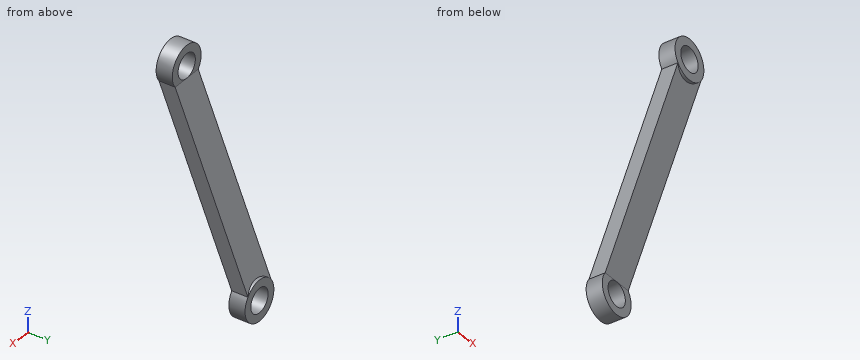
```python
from build123d import *

# Parameters (mm, degrees)
BOSS_EXTRUDE1_DEPTH = 4
SKETCH2_R           = 2.5
BOSS_EXTRUDE2_DEPTH = 2
SKETCH3_R           = 2.5
BOSS_EXTRUDE3_DEPTH = 2
SKETCH4_R           = 1.5
CUT_EXTRUDE1_DEPTH  = 28.879203719
SKETCH5_R           = 1.5
CUT_EXTRUDE2_DEPTH  = 29.587584718


with BuildPart() as part:
    # Sketch1 → Boss-Extrude1 (new body)
    with BuildSketch(Plane(origin=(0, 0, 0), x_dir=(0, 0, -1), z_dir=(1, 0, 0))):
        Polygon((0, 0), (0, 2), (22, 11), (22, 9), align=None)
    extrude(amount=BOSS_EXTRUDE1_DEPTH)

    # Sketch2 → Boss-Extrude2 (add)
    with BuildSketch(Plane(origin=(0, 0, 0), x_dir=(1, 0, 0), z_dir=(0, 1, 0))):
        with Locations((2, -1.5)):
            Circle(SKETCH2_R)
    extrude(amount=BOSS_EXTRUDE2_DEPTH)

    # Sketch3 → Boss-Extrude3 (add)
    with BuildSketch(Plane(origin=(0, 9, 0), x_dir=(-1, 0, 0), z_dir=(0, -1, 0))):
        with Locations((-2, 23.5)):
            Circle(SKETCH3_R)
    extrude(amount=-BOSS_EXTRUDE3_DEPTH)

    # Sketch4 → Cut-Extrude1 (cut, through all)
    with BuildSketch(Plane(origin=(0, 2, 0), x_dir=(1, 0, 0), z_dir=(0, 1, 0))):
        with Locations(Location((2, -1.5, 0), (0, 0, 270))):
            Circle(SKETCH4_R)
    extrude(amount=-CUT_EXTRUDE1_DEPTH, mode=Mode.SUBTRACT)

    # Sketch5 → Cut-Extrude2 (cut, through all)
    with BuildSketch(Plane(origin=(0, 11, 0), x_dir=(1, 0, 0), z_dir=(0, 1, 0))):
        with Locations(Location((2, 23.5, 0), (0, 0, 270))):
            Circle(SKETCH5_R)
    extrude(amount=-CUT_EXTRUDE2_DEPTH, mode=Mode.SUBTRACT)


solid = part.part
```
Read the model definition and answer for the solid it produces. Units are mm, in the model's axes. Round coordinates to 2 decimals unless told otherwise and drop trailing zeros. Write each loop counter-clockwise with the first axis right and the second up, starting at its lowest first coordinate (ties: lowest second). Pieces come first, ordered by that corner, then holes. Notation, with made-up numbers: M -39.75,-23 L -19.75,-23 A16 cw -19.75,-17 Z; hole C 50.25,3.5 d9. An arc over 180 degrees is marked long. One line per item, written item: value.
Q1. Flat-ended cylindrical pins translate along their axes: pin 1 Ø1.5 at (x, y) = (4, 4.5) entering from -Z; pin 2 Ø1.2 at (x, z) = (2.5, 1) entering from +Y; pin 3 Ø3 at (x, z) = (3.5, -15.5) entering from +Y; pin 4 Ø1.5 at (x, z) = (2.5, -1) entering from -Y. Find the tip coordinate at first contact, or state that the pin passes through.
Data:
pin 1: z = -12.83
pin 2: through
pin 3: y = 8.95
pin 4: y = 0
Q2. Find section C-C on y = 0.75. Write down the section's boundary in (x, z).
Data:
outline: M 0,-1.83 L 4,-1.83 L 4,0 A2.5 ccw long 0,0 Z; hole C 2,1.5 d3
Q3. Find section A-A on z = 1.5. Write down the section's boundary in (x, y).
Data:
outline: M -0.5,0 L 0.5,0 L 0.5,2 L -0.5,2 Z; M 3.5,0 L 4.5,0 L 4.5,2 L 3.5,2 Z
Q4. Find section B-B on x = 2.7. Write down the section's boundary in (y, z).
Data:
outline: M 0,-0.9 L 0.37,-0.9 L 9,-22 L 9,-22.17 L 11,-22.17 L 11,-21.1 L 10.63,-21.1 L 2,0 L 2,0.17 L 0,0.17 Z; M 0,2.83 L 2,2.83 L 2,3.9 L 0,3.9 Z; M 9,-25.9 L 11,-25.9 L 11,-24.83 L 9,-24.83 Z
Q5. Find section D-D on z = -16.25. Write down the section's boundary in (x, y).
Data:
outline: M 0,6.65 L 4,6.65 L 4,8.65 L 0,8.65 Z
Q6. Straight lines are drawn through the part: line 1 (Y direction, x = 3.85, z = -22.75); line 2 (X direction, y = 6.75, z = -14.5); line 3 (Z direction, x = 2, y = 0.9). For each, find the intervals that lie inside material, in ascending order. Write a range as [from, to].
Data:
line 1: [9, 11]
line 2: [0, 4]
line 3: [-2.2, 0], [3, 4]
